Part model, mm, in its own coordinate system. Round coordinates to 2 decimals unless told otherwise and drop trailing zeros. Loops run counter-clockwise (first coordinate to the right, second up) from the corner with the lowest first, then second, coordinate; pieces in that order, holes last. Notation, with made-up numbers: (80, 43) -> (123, 43) arc R5 ccw to (123, 52) -> close; hole circle Ø3 at (66, 72). An arc over 180 degrees is marked (long way). Answer as a JSON object with one key per item and string values. Group by question number.
from build123d import *

# Parameters (mm, degrees)
ESBO_O1_W                = 300
ESBO_O1_H                = 300
RESSALTO_EXTRUS_O1_DEPTH = 6
ESBO_O2_R                = 5
CORTE_EXTRUS_O1_DEPTH    = 213.216870206
ESBO_O3_R                = 12.5
CORTE_EXTRUS_O2_DEPTH    = 213.216870206


with BuildPart() as part:
    # Esboço1 → Ressalto-extrusão1 (new body)
    with BuildSketch(Plane(origin=(0, 0, 0), x_dir=(1, 0, 0), z_dir=(0, 1, 0))):
        Rectangle(ESBO_O1_W, ESBO_O1_H)
    extrude(amount=RESSALTO_EXTRUS_O1_DEPTH)

    # Esboço2 → Corte-extrusão1 (cut, through all)
    with BuildSketch(Plane(origin=(0, 6, 0), x_dir=(1, 0, 0), z_dir=(0, 1, 0))):
        with Locations(Location((-139, 139, 0), (0, 0, 270))):
            Circle(ESBO_O2_R)
        with Locations(Location((139, 139, 0), (0, 0, 270))):
            Circle(ESBO_O2_R)
        with Locations(Location((139, -139, 0), (0, 0, 270))):
            Circle(ESBO_O2_R)
        with Locations(Location((-139, -139, 0), (0, 0, 270))):
            Circle(ESBO_O2_R)
    extrude(amount=-CORTE_EXTRUS_O1_DEPTH, mode=Mode.SUBTRACT)

    # Esboço3 → Corte-extrusão2 (cut, through all)
    with BuildSketch(Plane(origin=(0, 6, 0), x_dir=(1, 0, 0), z_dir=(0, 1, 0))):
        with Locations(Location((-112, -112, 0), (0, 0, 270))):
            Circle(ESBO_O3_R)
        with Locations(Location((-80, -112, 0), (0, 0, 90))):
            Circle(ESBO_O3_R)
        with Locations(Location((-48, -112, 0), (0, 0, 270))):
            Circle(ESBO_O3_R)
        with Locations(Location((-16, -112, 0), (0, 0, 90))):
            Circle(ESBO_O3_R)
        with Locations(Location((16, -112, 0), (0, 0, 270))):
            Circle(ESBO_O3_R)
        with Locations(Location((48, -112, 0), (0, 0, 90))):
            Circle(ESBO_O3_R)
        with Locations(Location((80, -112, 0), (0, 0, 270))):
            Circle(ESBO_O3_R)
        with Locations(Location((112, -112, 0), (0, 0, 90))):
            Circle(ESBO_O3_R)
        with Locations(Location((112, -80, 0), (0, 0, 270))):
            Circle(ESBO_O3_R)
        with Locations(Location((80, -80, 0), (0, 0, 90))):
            Circle(ESBO_O3_R)
        with Locations(Location((48, -80, 0), (0, 0, 270))):
            Circle(ESBO_O3_R)
        with Locations(Location((16, -80, 0), (0, 0, 90))):
            Circle(ESBO_O3_R)
        with Locations(Location((-16, -80, 0), (0, 0, 270))):
            Circle(ESBO_O3_R)
        with Locations(Location((-48, -80, 0), (0, 0, 90))):
            Circle(ESBO_O3_R)
        with Locations(Location((-80, -80, 0), (0, 0, 270))):
            Circle(ESBO_O3_R)
        with Locations(Location((-112, -80, 0), (0, 0, 90))):
            Circle(ESBO_O3_R)
        with Locations(Location((112, -16, 0), (0, 0, 270))):
            Circle(ESBO_O3_R)
        with Locations(Location((112, -48, 0), (0, 0, 90))):
            Circle(ESBO_O3_R)
        with Locations(Location((80, -16, 0), (0, 0, 90))):
            Circle(ESBO_O3_R)
        with Locations(Location((80, -48, 0), (0, 0, 270))):
            Circle(ESBO_O3_R)
        with Locations(Location((48, -16, 0), (0, 0, 270))):
            Circle(ESBO_O3_R)
        with Locations(Location((48, -48, 0), (0, 0, 90))):
            Circle(ESBO_O3_R)
        with Locations(Location((16, -16, 0), (0, 0, 90))):
            Circle(ESBO_O3_R)
        with Locations(Location((16, -48, 0), (0, 0, 270))):
            Circle(ESBO_O3_R)
        with Locations(Location((-16, -16, 0), (0, 0, 270))):
            Circle(ESBO_O3_R)
        with Locations(Location((-16, -48, 0), (0, 0, 90))):
            Circle(ESBO_O3_R)
        with Locations(Location((-48, -16, 0), (0, 0, 90))):
            Circle(ESBO_O3_R)
        with Locations(Location((-48, -48, 0), (0, 0, 270))):
            Circle(ESBO_O3_R)
        with Locations(Location((-80, -16, 0), (0, 0, 270))):
            Circle(ESBO_O3_R)
        with Locations(Location((-80, -48, 0), (0, 0, 90))):
            Circle(ESBO_O3_R)
        with Locations(Location((-112, -48, 0), (0, 0, 270))):
            Circle(ESBO_O3_R)
        with Locations(Location((-112, -16, 0), (0, 0, 90))):
            Circle(ESBO_O3_R)
        with Locations(Location((-112, 16, 0), (0, 0, 270))):
            Circle(ESBO_O3_R)
        with Locations(Location((-80, 16, 0), (0, 0, 90))):
            Circle(ESBO_O3_R)
        with Locations(Location((-48, 16, 0), (0, 0, 270))):
            Circle(ESBO_O3_R)
        with Locations(Location((-16, 16, 0), (0, 0, 90))):
            Circle(ESBO_O3_R)
        with Locations(Location((16, 16, 0), (0, 0, 270))):
            Circle(ESBO_O3_R)
        with Locations(Location((48, 16, 0), (0, 0, 90))):
            Circle(ESBO_O3_R)
        with Locations(Location((80, 16, 0), (0, 0, 270))):
            Circle(ESBO_O3_R)
        with Locations(Location((112, 16, 0), (0, 0, 90))):
            Circle(ESBO_O3_R)
        with Locations(Location((112, 48, 0), (0, 0, 270))):
            Circle(ESBO_O3_R)
        with Locations(Location((80, 48, 0), (0, 0, 90))):
            Circle(ESBO_O3_R)
        with Locations(Location((48, 48, 0), (0, 0, 270))):
            Circle(ESBO_O3_R)
        with Locations(Location((16, 48, 0), (0, 0, 90))):
            Circle(ESBO_O3_R)
        with Locations(Location((-16, 48, 0), (0, 0, 270))):
            Circle(ESBO_O3_R)
        with Locations(Location((-48, 48, 0), (0, 0, 90))):
            Circle(ESBO_O3_R)
        with Locations(Location((-80, 48, 0), (0, 0, 270))):
            Circle(ESBO_O3_R)
        with Locations(Location((-112, 48, 0), (0, 0, 90))):
            Circle(ESBO_O3_R)
        with Locations(Location((-112, 80, 0), (0, 0, 270))):
            Circle(ESBO_O3_R)
        with Locations(Location((-80, 80, 0), (0, 0, 90))):
            Circle(ESBO_O3_R)
        with Locations(Location((-48, 80, 0), (0, 0, 270))):
            Circle(ESBO_O3_R)
        with Locations(Location((-16, 80, 0), (0, 0, 90))):
            Circle(ESBO_O3_R)
        with Locations(Location((16, 80, 0), (0, 0, 270))):
            Circle(ESBO_O3_R)
        with Locations(Location((48, 80, 0), (0, 0, 90))):
            Circle(ESBO_O3_R)
        with Locations(Location((80, 80, 0), (0, 0, 270))):
            Circle(ESBO_O3_R)
        with Locations(Location((112, 80, 0), (0, 0, 90))):
            Circle(ESBO_O3_R)
        with Locations(Location((112, 112, 0), (0, 0, 270))):
            Circle(ESBO_O3_R)
        with Locations(Location((80, 112, 0), (0, 0, 90))):
            Circle(ESBO_O3_R)
        with Locations(Location((48, 112, 0), (0, 0, 270))):
            Circle(ESBO_O3_R)
        with Locations(Location((16, 112, 0), (0, 0, 90))):
            Circle(ESBO_O3_R)
        with Locations(Location((-16, 112, 0), (0, 0, 270))):
            Circle(ESBO_O3_R)
        with Locations(Location((-48, 112, 0), (0, 0, 90))):
            Circle(ESBO_O3_R)
        with Locations(Location((-80, 112, 0), (0, 0, 270))):
            Circle(ESBO_O3_R)
        with Locations(Location((-112, 112, 0), (0, 0, 90))):
            Circle(ESBO_O3_R)
    extrude(amount=-CORTE_EXTRUS_O2_DEPTH, mode=Mode.SUBTRACT)


solid = part.part
Item 1: Two-plate mould, pull along X, no slides. Class faces 1 (the face through (-108.245, 3.042, 123.923)), 2 (the face through (-92.394, 3.042, -14.373)), 3 (the face through (-2, 6, -2)): pulls with the +X half, pulls with the -X half, needs draft (parallel to the pull), parting line crosses it, or undercut.
Item 2: Band-saw the part on B-B, the plane x = 48. Count the separate pieces of the cut face and the enclosed holes in it, plus the area to 3 significant figures.
Item 3: Band-saw the part on A-A, the plane z = -139. List the corners of the cut face in (x, y), plus the area to 3 significant figures.
Entries:
{
 "1": {"face 1": "undercut", "face 2": "undercut", "face 3": "needs draft"},
 "2": {"separate pieces": "9", "enclosed holes": "0", "area": "600 mm²"},
 "3": {"outline": "(-150, 0) -> (-144, 0) -> (-144, 6) -> (-150, 6) -> close; (-134, 0) -> (134, 0) -> (134, 6) -> (-134, 6) -> close; (144, 0) -> (150, 0) -> (150, 6) -> (144, 6) -> close", "area": "1,680 mm²"}
}
